Source: CAD feature listing. Evaluate the final solid. Frame: model axes, mm. Give positions to 0.01 mm unless a question says otherwise; leave off trailing zeros. Loops run counter-clockwise (first coordinate to the right, second up) from the corner with the lowest first, then second, coordinate; pieces in that order, holes last. Notation, with made-up numbers: M 34.5,-36.5 L 67.5,-36.5 A23 cw 67.5,-15.5 Z; hole C 56.5,25.25 d2. An arc over 180 degrees is marked long. Put each result on its own line as item: value.
from build123d import *

# Parameters (mm, degrees)
F0_W     = 6
F0_H     = 4.448176
F0_R     = 0.125
F0_R_2   = 0.065
F0_W_2   = 5
F1_DEPTH = 0.375


with BuildPart() as f1:
    # F0 (on Front) → F1 (new body)
    with BuildSketch(Plane.XZ):
        with Locations((-3, 0.120438)):
            Rectangle(F0_W, F0_H)
        with Locations((-5.5, -1)):
            Circle(F0_R, mode=Mode.SUBTRACT)
        with Locations((-2.283164, -1)):
            Circle(F0_R_2, mode=Mode.SUBTRACT)
        with Locations((-5.5, 1)):
            Circle(F0_R, mode=Mode.SUBTRACT)
        with Locations((-2.283164, 1)):
            Circle(F0_R_2, mode=Mode.SUBTRACT)
        with Locations((2.5, 0.120438)):
            Rectangle(F0_W_2, F0_H)
        with Locations((0.216836, -1)):
            Circle(F0_R_2, mode=Mode.SUBTRACT)
        with Locations((4, -1)):
            Circle(F0_R, mode=Mode.SUBTRACT)
        with Locations((0.216836, 1)):
            Circle(F0_R_2, mode=Mode.SUBTRACT)
        with Locations((4, 1)):
            Circle(F0_R, mode=Mode.SUBTRACT)
    extrude(amount=F1_DEPTH)


solid = f1.part
1. Material intervals for line 1 (Z direction, x = -5.5, y = -0.15) (3 decimals), sorted ascending. Write a range as from..to.
Found:
line 1: -2.104..-1.125, -0.875..0.875, 1.125..2.345
2. Section query A-A (x = 4). Output: boundary loops of the cut face in (y, z) (3 decimals), plus the area to 3 significant figures.
Found:
outline: M -0.375,-2.104 L 0,-2.104 L 0,-1.125 L -0.375,-1.125 Z; M -0.375,-0.875 L 0,-0.875 L 0,0.875 L -0.375,0.875 Z; M -0.375,1.125 L 0,1.125 L 0,2.345 L -0.375,2.345 Z
area: 1.48 mm^2
3. Draft query along Y for faces 1 (the flat face through (-1, -0.375, 0)), 2 (the flat face through (-1, 0, 0)). Return one class per face: pulls with the +Y half, pulls with the -Y half, needs draft (parallel to the pull), parting line crosses it, or undercut.
Found:
face 1: pulls with the -Y half
face 2: pulls with the +Y half
